Geometry check sheet. Reference: the model listing, model coordinates, mm. Give positions to 0.01 mm unless a question says otherwise; leave off trailing zeros. Order: outer loops, then holes, each group sorted by start corner. A loop starts at its lowest first (then second) coordinate and runs counter-clockwise, first axis right, second up. Notation, with made-up numbers: M 24.5,-4.5 L 82.5,-4.5 A9 cw 82.5,-0.5 Z; hole C 37,-6.75 d9. An arc over 180 degrees is marked long. Put each result on its own line as item: value. Start each with the question number.
Q1. Material ranges on L1, parallel to Y at x = 0, z = 4.75; L2, parallel to Y at x = 11.5, z = 3.5; L3, parallel to X at y = -6.5, z = 4.75, recorded low to high.
Q2. Section check A-A on y = 47.5. Record the cut outline in (x, z), then the cut area to 3 significant figures.
Q3. Go/stop test with flat-tipped pins: pin 1 (2 mm diameter, centred on y = 46.5, z = 4, fed in from -X); pin 2 (3 mm diameter, centred on y = 8.5, z = 5, fed in from +X); pin 3 (1.5 mm diameter, centred on x = 12.5, z = 4, fed in from -Y). Record where each tip stops, or that it passes through.
Q4. Section check B-B on x = 18.5. Record the cut outline in (y, z), then the cut area to 3 significant figures.
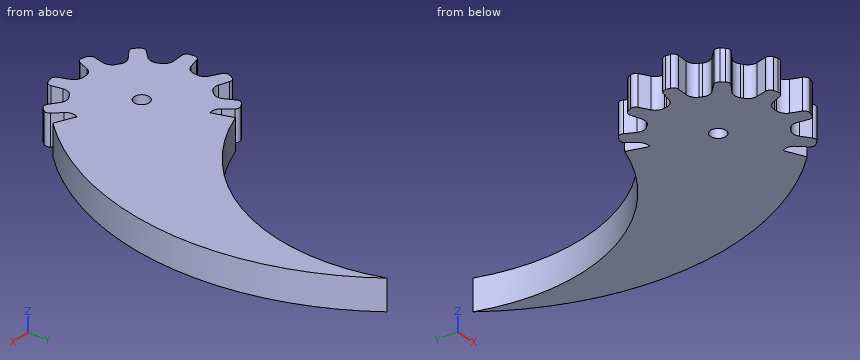
```python
from build123d import *

# Parameters (mm, degrees)
ESBO_O1_R                = 1.6
RESSALTO_EXTRUS_O1_DEPTH = 6.5
RESSALTO_EXTRUS_O2_DEPTH = 6.5


with BuildPart() as part:
    # Esboço1 → Ressalto-extrusão1 (new body)
    with BuildSketch(Plane.XY):
        with BuildLine():
            Line((7.237292739, 13.882644275), (5.840999253, 12.115479156))
            ThreePointArc((5.840999253, 12.115479156), (4.855639954, 11.442537909), (3.66244261, 11.450473127))
            ThreePointArc((3.66244261, 11.450473127), (3.390740604, 11.533850132), (3.117143568, 11.610781054))
            ThreePointArc((3.117143568, 11.610781054), (2.102970634, 12.257593135), (1.64323621, 13.369149192))
            Line((1.64323621, 13.369149192), (1.451023847, 15.579942687))
            ThreePointArc((1.451023847, 15.579942687), (1.141313879, 16.220426504), (0.484122849, 16.4928962))
            ThreePointArc((0.484122849, 16.4928962), (0.017522037, 16.499990696), (-0.449092791, 16.493887221))
            ThreePointArc((-0.449092791, 16.493887221), (-1.103704511, 16.225768855), (-1.417126065, 15.591599404))
            Line((-1.417126065, 15.591599404), (-1.636361298, 13.350072253))
            ThreePointArc((-1.636361298, 13.350072253), (-2.101478783, 12.251232594), (-3.109550367, 11.612816937))
            ThreePointArc((-3.109550367, 11.612816937), (-3.383197652, 11.536064942), (-3.654954122, 11.452865627))
            ThreePointArc((-3.654954122, 11.452865627), (-4.857823698, 11.448695291), (-5.845529481, 12.135244556))
            Line((-5.845529481, 12.135244556), (-7.202474013, 13.891164545))
            ThreePointArc((-7.202474013, 13.891164545), (-7.809290312, 14.262531969), (-8.509462826, 14.136443768))
            ThreePointArc((-8.509462826, 14.136443768), (-8.905827982, 13.890148593), (-9.295069567, 13.632743002))
            ThreePointArc((-9.295069567, 13.632743002), (-9.700808257, 13.053277663), (-9.621617356, 12.350331887))
            Line((-9.621617356, 12.350331887), (-8.594188699, 10.346111737))
            ThreePointArc((-8.594188699, 10.346111737), (-8.391392855, 9.170247495), (-8.894283074, 8.088173422))
            ThreePointArc((-8.894283074, 8.088173422), (-9.082994557, 7.875660644), (-9.266629702, 7.658746286))
            ThreePointArc((-9.266629702, 7.658746286), (-10.276293328, 7.004917585), (-11.478380864, 7.048485517))
            Line((-11.478380864, 7.048485517), (-13.569237263, 7.792039811))
            ThreePointArc((-13.569237263, 7.792039811), (-14.280500006, 7.776384308), (-14.80135418, 7.291770323))
            ThreePointArc((-14.80135418, 7.291770323), (-15.001640543, 6.870282455), (-15.189927432, 6.443299203))
            ThreePointArc((-15.189927432, 6.443299203), (-15.217973923, 5.736463043), (-14.771313119, 5.187921259))
            Line((-14.771313119, 5.187921259), (-12.823421912, 4.057333846))
            ThreePointArc((-12.823421912, 4.057333846), (-12.017098986, 3.177773609), (-11.855143748, 1.995591994))
            ThreePointArc((-11.855143748, 1.995591994), (-11.899004868, 1.714789737), (-11.936215827, 1.433029113))
            ThreePointArc((-11.936215827, 1.433029113), (-12.432112436, 0.33712804), (-13.466927425, -0.276117871))
            Line((-13.466927425, -0.276117871), (-15.627863558, -0.781002507))
            ThreePointArc((-15.627863558, -0.781002507), (-16.21775185, -1.178710425), (-16.393920163, -1.867988679))
            ThreePointArc((-16.393920163, -1.867988679), (-16.334538228, -2.330849819), (-16.262090664, -2.791846566))
            ThreePointArc((-16.262090664, -2.791846566), (-15.903540395, -3.401638061), (-15.231221337, -3.621617713))
            Line((-15.231221337, -3.621617713), (-12.981309273, -3.519618873))
            ThreePointArc((-12.981309273, -3.519618873), (-11.827461098, -3.823620944), (-11.052080047, -4.730575792))
            ThreePointArc((-11.052080047, -4.730575792), (-10.937165208, -4.990514794), (-10.816137764, -5.247664678))
            ThreePointArc((-10.816137764, -5.247664678), (-10.640823687, -6.437697275), (-11.179819681, -7.513055786))
            Line((-11.179819681, -7.513055786), (-12.724753595, -9.106082048))
            ThreePointArc((-12.724753595, -9.106082048), (-13.005982071, -9.759572927), (-12.781532328, -10.434674473))
            ThreePointArc((-12.781532328, -10.434674473), (-12.48133544, -10.791953745), (-12.171155012, -11.140600777))
            ThreePointArc((-12.171155012, -11.140600777), (-11.53984516, -11.459743115), (-10.855324398, -11.28131865))
            Line((-10.855324398, -11.28131865), (-9.017722662, -9.979117468))
            ThreePointArc((-9.017722662, -9.979117468), (-7.88268788, -9.611042864), (-6.740059022, -9.954819189))
            ThreePointArc((-6.740059022, -9.954819189), (-6.502852873, -10.11136614), (-6.262012384, -10.262262012))
            ThreePointArc((-6.262012384, -10.262262012), (-5.471148601, -11.168599193), (-5.343198182, -12.364651574))
            Line((-5.343198182, -12.364651574), (-5.781624274, -14.540044879))
            ThreePointArc((-5.781624274, -14.540044879), (-5.664904879, -15.241839982), (-5.111098288, -15.68842485))
            ThreePointArc((-5.111098288, -15.68842485), (-4.665396838, -15.826688609), (-4.215963642, -15.952292956))
            ThreePointArc((-4.215963642, -15.952292956), (-3.512330623, -15.879460702), (-3.032938663, -15.359280625))
            Line((-3.032938663, -15.359280625), (-2.191072822, -13.270316777))
            ThreePointArc((-2.191072822, -13.270316777), (-1.435216957, -12.347026583), (-0.28811688, -12.018477831))
            ThreePointArc((-0.28811688, -12.018477831), (-0.003930697, -12.02193018), (0.280257682, -12.018663667))
            ThreePointArc((0.280257682, -12.018663667), (1.435577508, -12.35354978), (2.189850988, -13.290557851))
            Line((2.189850988, -13.290557851), (2.997129903, -15.357646195))
            ThreePointArc((2.997129903, -15.357646195), (3.474739585, -15.884930537), (4.182073344, -15.961211187))
            ThreePointArc((4.182073344, -15.961211187), (4.631772295, -15.836561666), (5.077766396, -15.699244836))
            ThreePointArc((5.077766396, -15.699244836), (5.630324069, -15.257561714), (5.752383667, -14.560779526))
            Line((5.752383667, -14.560779526), (5.331227158, -12.348284272))
            ThreePointArc((5.331227158, -12.348284272), (5.46792521, -11.162916602), (6.255300336, -10.26635468))
            ThreePointArc((6.255300336, -10.26635468), (6.496239447, -10.11561633), (6.733547915, -9.959224527))
            ThreePointArc((6.733547915, -9.959224527), (7.886517902, -9.616335598), (9.027637941, -9.996805918))
            Line((9.027637941, -9.996805918), (10.824316513, -11.299303357))
            ThreePointArc((10.824316513, -11.299303357), (11.511178782, -11.484667883), (12.147466239, -11.166425748))
            ThreePointArc((12.147466239, -11.166425748), (12.458386452, -10.81843829), (12.759341481, -10.461797406))
            ThreePointArc((12.759341481, -10.461797406), (12.985390652, -9.791494687), (12.711364828, -9.139333809))
            Line((12.711364828, -9.139333809), (11.160900184, -7.505758759))
            ThreePointArc((11.160900184, -7.505758759), (10.635039757, -6.434659473), (10.812703893, -5.254736456))
            ThreePointArc((10.812703893, -5.254736456), (10.933899467, -4.99766577), (11.048984261, -4.737801968))
            ThreePointArc((11.048984261, -4.737801968), (11.833544585, -3.826002809), (12.999213634, -3.529138739))
            Line((12.999213634, -3.529138739), (15.21485911, -3.65351154))
            ThreePointArc((15.21485911, -3.65351154), (15.89290005, -3.438104324), (16.256124433, -2.826379032))
            ThreePointArc((16.256124433, -2.826379032), (16.329550936, -2.365537195), (16.389915799, -1.902803219))
            ThreePointArc((16.389915799, -1.902803219), (16.217687452, -1.21669728), (15.63457747, -0.816214183))
            Line((15.63457747, -0.816214183), (13.44706626, -0.280207874))
            ThreePointArc((13.44706626, -0.280207874), (12.425604324, 0.336556574), (11.937150363, 1.425223464))
            ThreePointArc((11.937150363, 1.425223464), (11.900123661, 1.707008361), (11.856446173, 1.987839239))
            ThreePointArc((11.856446173, 1.987839239), (12.023504475, 3.179058838), (12.843630847, 4.059005053))
            Line((12.843630847, 4.059005053), (14.774791444, 5.152244377))
            ThreePointArc((14.774791444, 5.152244377), (15.228737846, 5.700033066), (15.203577979, 6.411023056))
            ThreePointArc((15.203577979, 6.411023056), (15.016198378, 6.838405244), (14.816807657, 7.260317546))
            ThreePointArc((14.816807657, 7.260317546), (14.300983076, 7.744392916), (13.593922234, 7.766047679))
            Line((13.593922234, 7.766047679), (11.463883812, 7.034307031))
            ThreePointArc((11.463883812, 7.034307031), (10.271127314, 7.000918286), (9.271635936, 7.652685004))
            ThreePointArc((9.271635936, 7.652685004), (9.088142675, 7.869719398), (8.899570199, 8.082355534))
            ThreePointArc((8.899570199, 8.082355534), (8.396086648, 9.174791766), (8.610286014, 10.358443421))
            Line((8.610286014, 10.358443421), (9.643831887, 12.322199108))
            ThreePointArc((9.643831887, 12.322199108), (9.729558977, 13.028450232), (9.324002941, 13.612970622))
            ThreePointArc((9.324002941, 13.612970622), (8.935308934, 13.871202336), (8.539467774, 14.118338788))
            ThreePointArc((8.539467774, 14.118338788), (7.843817619, 14.246693081), (7.237292739, 13.882644275))
        make_face()
        Circle(ESBO_O1_R, mode=Mode.SUBTRACT)
    extrude(amount=RESSALTO_EXTRUS_O1_DEPTH)

    # Esboço6 → Ressalto-extrusão2 (add)
    with BuildSketch(Plane.XY.offset(6.5)):
        with BuildLine():
            ThreePointArc((19.721119128, 67.164555089), (17.980474936, 36.295868824), (-5.07780376, 15.699232751))
            Line((-5.07780376, 15.699232751), (-3.385202507, 10.466155167))
            ThreePointArc((-3.385202507, 10.466155167), (6.471582976, 8.894864461), (11, 0))
            ThreePointArc((11, 0), (10.747375274, -2.343912268), (10.001104596, -4.580164501))
            Line((10.001104596, -4.580164501), (15.001656894, -6.870246751))
            ThreePointArc((15.001656894, -6.870246751), (30.834620096, 29.288282282), (19.721119128, 67.164555089))
        make_face()
    extrude(amount=-RESSALTO_EXTRUS_O2_DEPTH)


solid = part.part
```
Results found:
1. L1: y = -12.02 to -1.6, 1.6 to 17.87
1. L2: y = -11.49 to -7.86, -5.27 to 26.68
1. L3: x = -10.65 to 10.65, 14.19 to 15.35
2. outline: M 21.49,0 L 29.09,0 L 29.09,6.5 L 21.49,6.5 Z
2. area: 49.4 mm^2
3. pin 1: stops at x = 21.12
3. pin 2: stops at x = 26.19
3. pin 3: stops at y = -11.43
4. outline: M -2.85,0 L 37.42,0 L 37.42,6.5 L -2.85,6.5 Z
4. area: 262 mm^2
